from build123d import *

# Parameters (mm, degrees)
SKETCH1_R           = 2
BOSS_EXTRUDE1_DEPTH = 3


with BuildPart() as part:
    # Sketch1 → Boss-Extrude1 (new body)
    with BuildSketch(Plane(origin=(0, 0, 0), x_dir=(-1, 0, 0), z_dir=(0, 0, -1))):
        with BuildLine():
            Line((-82.5, -212.5), (82.5, -212.5))
            ThreePointArc((82.5, -212.5), (87.803300859, -210.303300859), (90, -205))
            ThreePointArc((90, -205), (103.180194847, -173.180194847), (135, -160))
            ThreePointArc((135, -160), (140.303300859, -157.803300859), (142.5, -152.5))
            Line((142.5, -152.5), (142.5, 152.5))
            ThreePointArc((142.5, 152.5), (140.303300859, 157.803300859), (135, 160))
            ThreePointArc((135, 160), (103.180194847, 173.180194847), (90, 205))
            ThreePointArc((90, 205), (87.803300859, 210.303300859), (82.5, 212.5))
            Line((82.5, 212.5), (-82.5, 212.5))
            ThreePointArc((-82.5, 212.5), (-87.803300859, 210.303300859), (-90, 205))
            ThreePointArc((-90, 205), (-103.180194847, 173.180194847), (-135, 160))
            ThreePointArc((-135, 160), (-140.303300859, 157.803300859), (-142.5, 152.5))
            Line((-142.5, 152.5), (-142.5, -152.5))
            ThreePointArc((-142.5, -152.5), (-140.303300859, -157.803300859), (-135, -160))
            ThreePointArc((-135, -160), (-103.180194847, -173.180194847), (-90, -205))
            ThreePointArc((-90, -205), (-87.803300859, -210.303300859), (-82.5, -212.5))
        make_face()
        with Locations((-135, 20)):
            Circle(SKETCH1_R, mode=Mode.SUBTRACT)
        with Locations(Location((-135, -140, 0), (0, 0, 180))):
            Circle(SKETCH1_R, mode=Mode.SUBTRACT)
        with Locations(Location((-82.5, -205, 0), (0, 0, 180))):
            Circle(SKETCH1_R, mode=Mode.SUBTRACT)
        with Locations(Location((-6.25, -205, 0), (0, 0, 180))):
            Circle(SKETCH1_R, mode=Mode.SUBTRACT)
        with Locations((135, 20)):
            Circle(SKETCH1_R, mode=Mode.SUBTRACT)
        with Locations(Location((135, 140, 0), (0, 0, 180))):
            Circle(SKETCH1_R, mode=Mode.SUBTRACT)
        with Locations(Location((82.5, 205, 0), (0, 0, 180))):
            Circle(SKETCH1_R, mode=Mode.SUBTRACT)
        with Locations(Location((70, 205, 0), (0, 0, 180))):
            Circle(SKETCH1_R, mode=Mode.SUBTRACT)
        with Locations(Location((135, 152.5, 0), (0, 0, 180))):
            Circle(SKETCH1_R, mode=Mode.SUBTRACT)
        with Locations((135, 0)):
            Circle(SKETCH1_R, mode=Mode.SUBTRACT)
        with Locations((135, -20)):
            Circle(SKETCH1_R, mode=Mode.SUBTRACT)
        with Locations((-135, 0)):
            Circle(SKETCH1_R, mode=Mode.SUBTRACT)
        with Locations(Location((135, -140, 0), (0, 0, 180))):
            Circle(SKETCH1_R, mode=Mode.SUBTRACT)
        with Locations(Location((135, -152.5, 0), (0, 0, 180))):
            Circle(SKETCH1_R, mode=Mode.SUBTRACT)
        with Locations(Location((82.5, -205, 0), (0, 0, 180))):
            Circle(SKETCH1_R, mode=Mode.SUBTRACT)
        with Locations(Location((70, -205, 0), (0, 0, 180))):
            Circle(SKETCH1_R, mode=Mode.SUBTRACT)
        with Locations(Location((6.25, -205, 0), (0, 0, 180))):
            Circle(SKETCH1_R, mode=Mode.SUBTRACT)
        with Locations(Location((-70, -205, 0), (0, 0, 180))):
            Circle(SKETCH1_R, mode=Mode.SUBTRACT)
        with Locations(Location((-135, -152.5, 0), (0, 0, 180))):
            Circle(SKETCH1_R, mode=Mode.SUBTRACT)
        with Locations((-135, -20)):
            Circle(SKETCH1_R, mode=Mode.SUBTRACT)
        with Locations(Location((-135, 140, 0), (0, 0, 180))):
            Circle(SKETCH1_R, mode=Mode.SUBTRACT)
        with Locations(Location((6.25, 205, 0), (0, 0, 180))):
            Circle(SKETCH1_R, mode=Mode.SUBTRACT)
        with Locations(Location((-6.25, 205, 0), (0, 0, 180))):
            Circle(SKETCH1_R, mode=Mode.SUBTRACT)
        with Locations(Location((-70, 205, 0), (0, 0, 180))):
            Circle(SKETCH1_R, mode=Mode.SUBTRACT)
        with Locations(Location((-135, 152.5, 0), (0, 0, 180))):
            Circle(SKETCH1_R, mode=Mode.SUBTRACT)
        with Locations(Location((-82.5, 205, 0), (0, 0, 180))):
            Circle(SKETCH1_R, mode=Mode.SUBTRACT)
    extrude(amount=-BOSS_EXTRUDE1_DEPTH)


solid = part.part
For this review, take the finished solid that the model builds, in its own axes (mm). Coordinates: 2 decimals unless noted, no trailing zeros. Order: outer loops, then holes, each group sorted by start corner. A loop starts at its lowest first (then second) coordinate and runs counter-clockwise, first axis right, second up. Notation, with made-up numbers: (10, 42) -> (24, 42) arc R26 ccw to (24, 57) -> close; hole circle Ø5 at (25, -17.75). An arc over 180 degrees is marked (long way). Return JSON: item names as keys, results as strings.
1. For line 1 (X direction, y = 140, z = 1.45); line 2 (Y direction, x = 82.5, z = 2.3); line 3 (X direction, y = -141.5, z = 1.1), list the stretches that pass through material, from the lowest coordinate up. Write a range as from..to.
Answer block:
{"line 1": "-142.5..-137, -133..133, 137..142.5", "line 2": "-212.5..-207, -203..203, 207..212.5", "line 3": "-142.5..-136.32, -133.68..133.68, 136.32..142.5"}
2. We need section A-A on z = 2.3. State how many separate pieces and enclosed holes the cut face has, and give its area (3 significant figures).
Answer block:
{"separate pieces": "1", "enclosed holes": "26", "area": "111,000 mm²"}
3. We need section C-C on x = 105. Write out the cut boundary in (y, z), and give its area (3 significant figures).
Answer block:
{"outline": "(-171.46, 0) -> (171.46, 0) -> (171.46, 3) -> (-171.46, 3) -> close", "area": "1,030 mm²"}
4. We need section B-B on x = -125. Write out the cut boundary in (y, z).
Answer block:
{"outline": "(-161.13, 0) -> (161.13, 0) -> (161.13, 3) -> (-161.13, 3) -> close"}
